CAD build for the part. Positions are in the model's coordinates, mm. A direction names the side the tool comes from. Round coordinates to 2 decimals unless told otherwise and drop trailing zeros. Loops run counter-clockwise (first coordinate to the right, second up) from the corner with the lowest first, then second, coordinate; pieces in that order, holes last. Notation, with made-up numbers: M 77,3.25 L 117,3.25 A25 cw 117,24.25 Z; hole C 78,43 d4. An arc over 180 degrees is marked long. Use one line per item in the form item = value.
from build123d import *

# Parameters (mm, degrees)
F1_DEPTH = 6.985
F2_R     = 1.016


with BuildPart() as f1:
    # F0 (on Top) → F1 (new body)
    with BuildSketch(Plane.XY):
        with BuildLine():
            ThreePointArc((-28.549569621, 1.114534499), (-18.8062884316, 10.8578156884), (-15.24, 24.1673853094))
            Line((-15.24, 24.1673853094), (-15.24, 36.7926146906))
            ThreePointArc((-15.24, 36.7926146906), (-24.3357044661, 14.0502255244), (-39.4833389937, -5.1980801916))
            Line((-39.4833389937, -5.1980801916), (-28.549569621, 1.114534499))
        make_face()
        with BuildLine():
            Line((15.24, 36.7926146906), (15.24, 24.1673853094))
            ThreePointArc((15.24, 24.1673853094), (18.8062884316, 10.8578156884), (28.549569621, 1.114534499))
            Line((28.549569621, 1.114534499), (39.4833389937, -5.1980801916))
            ThreePointArc((39.4833389937, -5.1980801916), (24.3357044661, 14.0502255244), (15.24, 36.7926146906))
        make_face()
        with BuildLine():
            Line((24.2433389937, -31.594534499), (13.309569621, -25.2819198084))
            ThreePointArc((13.309569621, -25.2819198084), (0, -21.7156313768), (-13.309569621, -25.2819198084))
            Line((-13.309569621, -25.2819198084), (-24.2433389937, -31.594534499))
            ThreePointArc((-24.2433389937, -31.594534499), (0, -28.1004510488), (24.2433389937, -31.594534499))
        make_face()
        Polygon((-6.3126146906, 15.24), (0, 15.24), (6.3126146906, 15.24), (15.24, 24.1673853094), (15.24, 36.7926146906), (6.3126146906, 45.72), (-6.3126146906, 45.72), (-15.24, 36.7926146906), (-15.24, 24.1673853094), align=None)
        with BuildLine():
            ThreePointArc((11.0109, 30.48), (7.785882057, 22.694117943), (0, 19.4691))
            ThreePointArc((0, 19.4691), (-7.785882057, 38.265882057), (11.0109, 30.48))
        make_face(mode=Mode.SUBTRACT)
        Polygon((-10.0419198084, -13.0868846863), (-13.1982271537, -7.62), (-16.354534499, -2.1531153137), (-28.549569621, 1.114534499), (-39.4833389937, -5.1980801916), (-42.7509888063, -17.3931153137), (-36.4383741157, -28.3268846863), (-24.2433389937, -31.594534499), (-13.309569621, -25.2819198084), align=None)
        with BuildLine():
            ThreePointArc((-15.3855543073, -15.24), (-37.032166988, -18.0898306237), (-16.8607351888, -9.73455))
            ThreePointArc((-16.8607351888, -9.73455), (-15.7607416267, -12.3901693763), (-15.3855543073, -15.24))
        make_face(mode=Mode.SUBTRACT)
        Polygon((16.354534499, -2.1531153137), (13.1982271537, -7.62), (10.0419198084, -13.0868846863), (13.309569621, -25.2819198084), (24.2433389937, -31.594534499), (36.4383741157, -28.3268846863), (42.7509888063, -17.3931153137), (39.4833389937, -5.1980801916), (28.549569621, 1.114534499), align=None)
        with BuildLine():
            ThreePointArc((37.4073543073, -15.24), (23.5466236836, -25.8757126807), (16.8607351888, -9.73455))
            ThreePointArc((16.8607351888, -9.73455), (29.2462849311, -4.6042873193), (37.4073543073, -15.24))
        make_face(mode=Mode.SUBTRACT)
        with BuildLine():
            ThreePointArc((-9.5357191185, -5.50545), (-9.5357191185, 5.50545), (0, 11.0109))
            Line((0, 11.0109), (0, 15.24))
            Line((0, 15.24), (-6.3126146906, 15.24))
            ThreePointArc((-6.3126146906, 15.24), (-16.354534499, 9.4422948954), (-16.354534499, -2.1531153137))
            Line((-16.354534499, -2.1531153137), (-13.1982271537, -7.62))
            Line((-13.1982271537, -7.62), (-9.5357191185, -5.50545))
        make_face()
        with BuildLine():
            ThreePointArc((0, 11.0109), (7.785882057, 7.785882057), (11.0109, 0))
            ThreePointArc((11.0109, 0), (10.6357126807, -2.8498306237), (9.5357191185, -5.50545))
            Line((9.5357191185, -5.50545), (13.1982271537, -7.62))
            Line((13.1982271537, -7.62), (16.354534499, -2.1531153137))
            ThreePointArc((16.354534499, -2.1531153137), (16.354534499, 9.4422948954), (6.3126146906, 15.24))
            Line((6.3126146906, 15.24), (0, 15.24))
            Line((0, 15.24), (0, 11.0109))
        make_face()
        with BuildLine():
            Line((13.1982271537, -7.62), (9.5357191185, -5.50545))
            ThreePointArc((9.5357191185, -5.50545), (0, -11.0109), (-9.5357191185, -5.50545))
            Line((-9.5357191185, -5.50545), (-13.1982271537, -7.62))
            Line((-13.1982271537, -7.62), (-10.0419198084, -13.0868846863))
            ThreePointArc((-10.0419198084, -13.0868846863), (0, -18.8845897909), (10.0419198084, -13.0868846863))
            Line((10.0419198084, -13.0868846863), (13.1982271537, -7.62))
        make_face()
    extrude(amount=F1_DEPTH)

    # F2#2 (call 1 of 2: OpenCascade refuses the feature's edges together)
    f2_2_edges = [f1.edges().sort_by_distance(p)[0] for p in [
        (0, -28.100451, 0),
        (-24.335704, 14.050226, 0),
        (24.335704, 14.050226, 0),
        (10.776307, 41.256307, 0),
        (0, 45.72, 0),
        (-10.776307, 41.256307, 0),
        (-30.340857, -29.96071, 0),
        (-39.594681, -22.86, 0),
        (-41.117164, -11.295598, 0),
        (30.340857, -29.96071, 0),
        (39.594681, -22.86, 0),
        (41.117164, -11.295598, 0),
    ]]
    fillet(f2_2_edges, radius=F2_R)

    # F2 (call 2 of 2)
    f2_edges = [f1.edges().sort_by_distance(p)[0] for p in [
        (0, -28.100451, 6.985),
        (-24.335704, 14.050226, 6.985),
        (24.335704, 14.050226, 6.985),
        (-10.776307, 41.256307, 6.985),
        (0, 45.72, 6.985),
        (10.776307, 41.256307, 6.985),
        (-39.594681, -22.86, 6.985),
        (-30.340857, -29.96071, 6.985),
        (-41.117164, -11.295598, 6.985),
        (30.340857, -29.96071, 6.985),
        (39.594681, -22.86, 6.985),
        (41.117164, -11.295598, 6.985),
    ]]
    fillet(f2_edges, radius=F2_R)


solid = f1.part
1. Pull direction X, two halves, no side cores. Call faces 3 (the face through (11.653, -19.099, 3.444)), 4 (the face through (-10.71, 41.32, 3.46)), 5 (the face through (39.55, -22.94, 3.46)): +X half, -X half, draft (parallel to the pull), parting line (faces both ways), or undercut.
Completed:
face_3 = undercut
face_4 = -X half
face_5 = +X half
2. Probe line 1 along Y through (x, z) = (-1, 2.25); line 2 along X through (y, z) = (3, 5); line 3 along Y through (x, z) = (19.5, 1.25). List the from-to ranges inside material, lowest first. Write a range as from..to.
Completed:
line_1 = -28.11..-21.73, -18.84..-10.97, 10.97..19.51, 41.45..45.72
line_2 = -31.92..-25.72, -17.89..-10.59, 10.59..17.89, 25.72..31.92
line_3 = -30.34..-23.82, -6.66..-1.31, 9.72..23.81
3. Cut at B-B on x = -4.5. State how many separate pieces and enclosed holes the cut face has, and give its area (3 significant figures).
Completed:
separate_pieces = 4
enclosed_holes = 0
area = 206 mm2
4. Drop flat-ended pins along their axis: P1, Ø2, axis at y = -13.5, z = 6, coming from the +X side; P2, Ø4, axis at x = 33.5, z = 2, coming from the -Y side; P3, Ø1, axis at x = -4, z = 6, coming from the -Y side; P4, Ø1.5, axis at x = 31.5, y = -23.5, coming from the +Z side. Give the stop position or say it passes through.
Completed:
P1 = 41.98
P2 = -29.65
P3 = -28.22
P4 = through
5. Tool access for faces 1 (the face through (-11.7, -19.27, 3.44)), 2 (the face through (-24.164, 14.349, 3.458)): list every direction of +Z, -Z, +X, -X, +Y, -Y with a clear straight run to the whole face (end or side of a thin tool).
Completed:
face_1 = +Z, -Z
face_2 = +Z, -Z, -X, +Y
6. Cut at A-A on z = 4.75. Write the cut outline in (x, y), and give its area (3 significant figures).
Completed:
outline = M -42.75,-17.39 L -36.44,-28.33 L -24.24,-31.59 A85.85 cw 24.24,-31.59 L 36.44,-28.33 L 42.75,-17.39 L 39.48,-5.2 A85.85 cw 15.24,36.79 L 6.31,45.72 L -6.31,45.72 L -15.24,36.79 A85.85 cw -39.48,-5.2 Z; hole C -26.4,-15.24 d22.02; hole M -28.55,1.11 L -16.35,-2.15 A11.6 cw -6.31,15.24 L -15.24,24.17 A26.62 cw Z; hole M -13.31,-25.28 A26.62 cw 13.31,-25.28 L 10.04,-13.09 A11.6 cw -10.04,-13.09 Z; hole C 0,0 d22.02; hole C 0,30.48 d22.02; hole M 6.31,15.24 A11.6 cw 16.35,-2.15 L 28.55,1.11 A26.62 cw 15.24,24.17 Z; hole C 26.4,-15.24 d22.02
area = 2,280 mm2
